Check sheet for the modelled part. Datum: model origin and axes. Units: mm. A direction names the side the tool comes from. Round coordinates to 2 decimals unless told otherwise and drop trailing zeros. Order: outer loops, then holes, each group sorted by start corner. A loop starts at its lowest first (then second) coordinate and runs counter-clockwise, first axis right, second up. Notation, with made-up numbers: (40.5, 17.25) -> (92.5, 17.25) arc R29 cw to (92.5, 44.25) -> close; hole circle Ø5 at (30.25, 67.25). An arc over 180 degrees is marked (long way). Answer in a Markdown table with one row per item.
```python
from build123d import *

# Parameters (mm, degrees)
SZKIC1_W                                          = 230
SZKIC1_H                                          = 242
DODANIE_WYCI_GNI_CIE1_DEPTH                       = 5
DODANIE_WYCI_GNI_CIE2_DEPTH                       = 145
SFAZOWANIE1_START                                 = -115
SFAZOWANIE1_DEPTH                                 = 116
SFAZOWANIE2_SIZE                                  = 10
SFAZOWANIE3_START                                 = -100
SFAZOWANIE3_DEPTH                                 = 210
POG_BIENIE_WALCOWE_POD_M3_RUB_Z_BEM_S_D           = 3.6
POG_BIENIE_WALCOWE_POD_M3_RUB_Z_BEM_S_DEPTH       = 6.7
POG_BIENIE_WALCOWE_POD_M3_RUB_Z_BEM_S_CBORE_D     = 7
POG_BIENIE_WALCOWE_POD_M3_RUB_Z_BEM_S_CBORE_DEPTH = 2.4
POG_BIENIE_WALCOWE_POD_M3_RUB_Z_BEM_S_TIP         = 1.081549114
POG_BIENIE_WALCOWE_POD_M3_RUB_Z_B_2_D             = 3.6
POG_BIENIE_WALCOWE_POD_M3_RUB_Z_B_2_DEPTH         = 6.7
POG_BIENIE_WALCOWE_POD_M3_RUB_Z_B_2_CBORE_D       = 7
POG_BIENIE_WALCOWE_POD_M3_RUB_Z_B_2_CBORE_DEPTH   = 2.4
POG_BIENIE_WALCOWE_POD_M3_RUB_Z_B_2_TIP           = 1.081549114
POG_BIENIE_WALCOWE_POD_M3_RUB_Z_B_3_D             = 3.6
POG_BIENIE_WALCOWE_POD_M3_RUB_Z_B_3_DEPTH         = 6.7
POG_BIENIE_WALCOWE_POD_M3_RUB_Z_B_3_CBORE_D       = 7
POG_BIENIE_WALCOWE_POD_M3_RUB_Z_B_3_CBORE_DEPTH   = 2.4
POG_BIENIE_WALCOWE_POD_M3_RUB_Z_B_3_TIP           = 1.081549114
SZKIC13_W                                         = 10
SZKIC13_H                                         = 7
DODANIE_WYCI_GNI_CIE3_DEPTH                       = 115
OTWORY_USTALAJ_CE_4_0MM1_D                        = 4
OTWORY_USTALAJ_CE_4_0MM1_DEPTH                    = 6.7
SFAZOWANIE4_SIZE                                  = 10


with BuildPart() as part:
    # Szkic1 → Dodanie-wyciągnięcie1 (new body)
    with BuildSketch(Plane.XY):
        Rectangle(SZKIC1_W, SZKIC1_H)
    extrude(amount=DODANIE_WYCI_GNI_CIE1_DEPTH)

    # Szkic6 → Dodanie-wyciągnięcie2 (add)
    with BuildSketch(Plane(origin=(0, 0, 0), x_dir=(-1, 0, 0), z_dir=(0, 0, -1))):
        Polygon((-115, 121), (-115, -121), (-110, -121), (-110, -116), (-110, 116), (110, 116), (115, 116), (115, 121), align=None)
    extrude(amount=DODANIE_WYCI_GNI_CIE2_DEPTH)

    # Sfazowanie1: read off the stored shape, not the designer's step
    # Sfazowanie1 outline → Sfazowanie1 (add)
    with BuildSketch(Plane.XY.offset(SFAZOWANIE1_START)):
        Polygon((110, 116), (100, 116), (110, 106), align=None)
    extrude(amount=SFAZOWANIE1_DEPTH)

    # Sfazowanie2
    sfazowanie2_edges = [part.edges().sort_by_distance(p)[0] for p in [
        (110, -7.5, 0),
        (105, 111, 0),
    ]]
    chamfer(sfazowanie2_edges, length=SFAZOWANIE2_SIZE)

    # Sfazowanie3: read off the stored shape, not the designer's step
    # Sfazowanie3 outline → Sfazowanie3 (add)
    with BuildSketch(Plane.YZ.offset(SFAZOWANIE3_START)):
        Polygon((106, 0), (116, -10), (116, 0), align=None)
    extrude(amount=SFAZOWANIE3_DEPTH)

    # Pog_bienie walcowe pod M3 _rub_ z _bem s
    with Locations(Plane(origin=(0, 121, 0), x_dir=(1, 0, 0), z_dir=(0, 1, 0))):
        with Locations((-76.666666667, 140), (-38.333333337, 140), (-7e-09, 140), (38.333333323, 140), (76.666666653, 140)):
            CounterBoreHole(POG_BIENIE_WALCOWE_POD_M3_RUB_Z_BEM_S_D / 2, POG_BIENIE_WALCOWE_POD_M3_RUB_Z_BEM_S_CBORE_D / 2, POG_BIENIE_WALCOWE_POD_M3_RUB_Z_BEM_S_CBORE_DEPTH, depth=POG_BIENIE_WALCOWE_POD_M3_RUB_Z_BEM_S_DEPTH)
            with Locations((0, 0, -(POG_BIENIE_WALCOWE_POD_M3_RUB_Z_BEM_S_DEPTH + POG_BIENIE_WALCOWE_POD_M3_RUB_Z_BEM_S_TIP / 2))):  # 118° drill point
                Cone(0, POG_BIENIE_WALCOWE_POD_M3_RUB_Z_BEM_S_D / 2, POG_BIENIE_WALCOWE_POD_M3_RUB_Z_BEM_S_TIP, mode=Mode.SUBTRACT)

    # Pog_bienie walcowe pod M3 _rub_ z _b 2
    with Locations(Plane(origin=(115, 0, 0), x_dir=(0, 0, -1), z_dir=(1, 0, 0))):
        with Locations((140, 80.666666667), (140, 40.333333337), (140, 7e-09), (140, -40.333333323), (140, -80.666666653)):
            CounterBoreHole(POG_BIENIE_WALCOWE_POD_M3_RUB_Z_B_2_D / 2, POG_BIENIE_WALCOWE_POD_M3_RUB_Z_B_2_CBORE_D / 2, POG_BIENIE_WALCOWE_POD_M3_RUB_Z_B_2_CBORE_DEPTH, depth=POG_BIENIE_WALCOWE_POD_M3_RUB_Z_B_2_DEPTH)
            with Locations((0, 0, -(POG_BIENIE_WALCOWE_POD_M3_RUB_Z_B_2_DEPTH + POG_BIENIE_WALCOWE_POD_M3_RUB_Z_B_2_TIP / 2))):  # 118° drill point
                Cone(0, POG_BIENIE_WALCOWE_POD_M3_RUB_Z_B_2_D / 2, POG_BIENIE_WALCOWE_POD_M3_RUB_Z_B_2_TIP, mode=Mode.SUBTRACT)

    # Pog_bienie walcowe pod M3 _rub_ z _b 3
    with Locations(Plane(origin=(0, 121, 0), x_dir=(1, 0, 0), z_dir=(0, 1, 0))):
        with Locations((-105, 105), (-105, 67.5), (-105, 35)):
            CounterBoreHole(POG_BIENIE_WALCOWE_POD_M3_RUB_Z_B_3_D / 2, POG_BIENIE_WALCOWE_POD_M3_RUB_Z_B_3_CBORE_D / 2, POG_BIENIE_WALCOWE_POD_M3_RUB_Z_B_3_CBORE_DEPTH, depth=POG_BIENIE_WALCOWE_POD_M3_RUB_Z_B_3_DEPTH)
            with Locations((0, 0, -(POG_BIENIE_WALCOWE_POD_M3_RUB_Z_B_3_DEPTH + POG_BIENIE_WALCOWE_POD_M3_RUB_Z_B_3_TIP / 2))):  # 118° drill point
                Cone(0, POG_BIENIE_WALCOWE_POD_M3_RUB_Z_B_3_D / 2, POG_BIENIE_WALCOWE_POD_M3_RUB_Z_B_3_TIP, mode=Mode.SUBTRACT)

    # Szkic13 → Dodanie-wyciągnięcie3 (add)
    with BuildSketch(Plane(origin=(0, 0, 0), x_dir=(-1, 0, 0), z_dir=(0, 0, -1))):
        with Locations((-105, -117.5)):
            Rectangle(SZKIC13_W, SZKIC13_H)
    extrude(amount=DODANIE_WYCI_GNI_CIE3_DEPTH)

    # Otwory ustalające Ø4.0mm1
    with Locations(Plane.XZ.offset(121)):
        with Locations((105, -105), (105, -67.5), (105, -35)):
            Hole(OTWORY_USTALAJ_CE_4_0MM1_D / 2, depth=OTWORY_USTALAJ_CE_4_0MM1_DEPTH)

    # Sfazowanie4
    sfazowanie4_edges = [part.edges().sort_by_distance(p)[0] for p in [
        (110, -117.5, -115),
        (110, -114, -62.5),
    ]]
    chamfer(sfazowanie4_edges, length=SFAZOWANIE4_SIZE - 0.0001)  # a hair under: the kernel refuses the full size


solid = part.part
```
(1) Tool access check on faces 4 (the flat face through (112.6, 1, -138)), 5 (the flat face through (38, 118.6, -142)), 6 (the flat face through (102.27, 108.13, -6.04)), 7 (the flat face through (-9, -1, 0)). Record the directions out of +Z, -Z, +X, -X, +Y, -Y that give a thin tool (end or side, any length) a straight path to the whole face; none if there is none.
Solutions:
| item | result |
|---|---|
| face 4 | +X |
| face 5 | +Y |
| face 6 | -Z, -X |
| face 7 | -Z, -X, -Y |
(2) Draft check along Z on faces 1 (the flat face through (111, 54, -145)), 2 (the flat face through (100, -118, -57)), 3 (the cylindrical face through (-101.66, 119.82, -36.05)). Enter one of: pulls with the +Z half, pulls with the -Z half, needs draft (parallel to the pull), parting line crosses it, or undercut.
Solutions:
| item | result |
|---|---|
| face 1 | pulls with the -Z half |
| face 2 | needs draft |
| face 3 | undercut |
(3) Section check A-A on y = 88.5. Record the boundary of the cut face in (x, z).
Solutions:
| item | result |
|---|---|
| outline | (-115, 0) -> (100, 0) -> (110, -10) -> (110, -145) -> (115, -145) -> (115, 5) -> (-115, 5) -> close |
(4) Scan lines: probe 1 along Z at (x, y) = (-105, 116.9); probe 2 along X at (y, z) = (119, -140); probe 3 along Y at (x, z) = (110.5, -140). Record each from-to range of solid material in increasing order. Write a range as from..to.
Solutions:
| item | result |
|---|---|
| probe 1 | -145..-106.8, -103.2..-69.3, -65.7..-36.8, -33.2..5 |
| probe 2 | -115..-80.17, -73.17..-41.83, -34.83..-3.5, 3.5..34.83, 41.83..73.17, 80.17..115 |
| probe 3 | -121..-82.47, -78.87..-42.13, -38.53..-1.8, 1.8..38.53, 42.13..78.87, 82.47..121 |
(5) Section check B-B on z = -131. Record the boundary of the cut face in (x, y).
Solutions:
| item | result |
|---|---|
| outline | (-115, 116) -> (110, 116) -> (110, -121) -> (115, -121) -> (115, 121) -> (-115, 121) -> close |
(6) Section check C-C on x = -12.5. Record the boundary of the cut face in (y, z), plus the area to 4 significant figures.
Solutions:
| item | result |
|---|---|
| outline | (-121, 0) -> (106, 0) -> (116, -10) -> (116, -145) -> (121, -145) -> (121, 5) -> (-121, 5) -> close |
| area | 1,985 mm^2 |
(7) Depth check by flat-ended pin: pin 1 Ø2.5 at (x, z) = (105, -35) entering from -Y; pin 2 Ø10 at (x, y) = (-53.5, -90) entering from -Z; pin 3 Ø9 at (x, z) = (-105, -35) entering from -Y. Enter the tip coordinate at first touch or a pass-through.
Solutions:
| item | result |
|---|---|
| pin 1 | y = -114.3 |
| pin 2 | z = 0 |
| pin 3 | y = 116 |
